from build123d import *

# Parameters (mm, degrees)
SKETCH1_W           = 26.25
SKETCH1_H           = 22
SKETCH1_R           = 3
SKETCH1_R_2         = 13
BOSS_EXTRUDE1_DEPTH = 5
FILLET1_R           = 5
SKETCH2_R           = 1.625
CUT_EXTRUDE1_DEPTH  = 5
CUT_EXTRUDE2_START  = -5
SKETCH3_R           = 1.15
SKETCH3_R_2         = 13
CUT_EXTRUDE2_DEPTH  = 5
SKETCH5_W           = 20
SKETCH5_H           = 3
BOSS_EXTRUDE2_DEPTH = 10
SKETCH6_R           = 1.65
CUT_EXTRUDE4_DEPTH  = 28
CHAMFER1_SIZE       = 10
CHAMFER1_SIZE_2     = 17.320508076
SKETCH9_W           = 20
SKETCH9_H           = 5
CUT_EXTRUDE6_DEPTH  = 5
FILLET3_R           = 5
CUT_EXTRUDE9_START  = -3
CUT_EXTRUDE9_DEPTH  = 3
SKETCH16_W          = 40
SKETCH16_H          = 8
CUT_EXTRUDE11_DEPTH = 10
SKETCH17_W          = 88.86330123
SKETCH17_H          = 4
CUT_EXTRUDE12_DEPTH = 10


# Some blends are built 0.0001 mm under size
with BuildPart() as part:
    # Sketch1 → Boss-Extrude1 (new body)
    # profile 1 of 3: a face of its own
    with BuildSketch(Plane(origin=(0, 0, 0), x_dir=(1, 0, 0), z_dir=(0, 1, 0))):
        with Locations((18.375, 0)):
            Rectangle(SKETCH1_W, SKETCH1_H)
        with Locations(Location((20, 0, 0), (0, 0, 270))):
            Circle(SKETCH1_R, mode=Mode.SUBTRACT)
    # profile 2 of 3: a face of its own
    with BuildSketch(Plane(origin=(0, 0, 0), x_dir=(1, 0, 0), z_dir=(0, 1, 0))):
        with Locations((-18.375, 0)):
            Rectangle(SKETCH1_W, SKETCH1_H)
        with Locations(Location((-20, 0, 0), (0, 0, 270))):
            Circle(SKETCH1_R, mode=Mode.SUBTRACT)
    # profile 3 of 3: a face of its own
    with BuildSketch(Plane(origin=(0, 0, 0), x_dir=(1, 0, 0), z_dir=(0, 1, 0))):
        with BuildLine():
            Line((-5.25, -11), (-31.5, -11))
            Line((-31.5, -11), (-50, -11))
            add(Edge.make_bspline(
                [(-50, -11), (-77.2307176, -35.658609428), (-60, -76)],
                knots=[0, 0, 0, 1, 1, 1], degree=2))
            Line((-60, -76), (-22, -76))
            Line((-22, -76), (-22, -51))
            Line((-22, -51), (22, -51))
            Line((22, -51), (22, -76))
            Line((22, -76), (60, -76))
            add(Edge.make_bspline(
                [(50, -11), (77.2307176, -35.658609428), (60, -76)],
                knots=[0, 0, 0, 1, 1, 1], degree=2))
            Line((50, -11), (31.5, -11))
            Line((31.5, -11), (5.25, -11))
            Line((5.25, -11), (-5.25, -11))
        make_face()
        with Locations(Location((-38, -60, 0), (0, 0, 270))):
            Circle(SKETCH1_R_2, mode=Mode.SUBTRACT)
        with Locations(Location((38, -60, 0), (0, 0, 270))):
            Circle(SKETCH1_R_2, mode=Mode.SUBTRACT)
    extrude(amount=BOSS_EXTRUDE1_DEPTH)

    # Fillet1
    fillet1_edges = [part.edges().sort_by_distance(p)[0] for p in [
        (60, 2.5, 76),
        (-60, 2.5, 76),
    ]]
    fillet(fillet1_edges, radius=FILLET1_R)

    # Sketch2 → Cut-Extrude1 (cut)
    with BuildSketch(Plane(origin=(0, 5, 0), x_dir=(1, 0, 0), z_dir=(0, 1, 0))):
        with Locations(Location((-60, -56, 0), (0, 0, 270))):
            Circle(SKETCH2_R)
        with Locations(Location((60, -56, 0), (0, 0, 270))):
            Circle(SKETCH2_R)
        with Locations(Location((-45, -17, 0), (0, 0, 270))):
            Circle(SKETCH2_R)
        with Locations(Location((-60, -34, 0), (0, 0, 270))):
            Circle(SKETCH2_R)
        with Locations(Location((60, -34, 0), (0, 0, 270))):
            Circle(SKETCH2_R)
        with Locations(Location((45, -17, 0), (0, 0, 270))):
            Circle(SKETCH2_R)
        with Locations(Location((0, -18, 0), (0, 0, 270))):
            Circle(SKETCH2_R)
        with Locations(Location((0, -36, 0), (0, 0, 270))):
            Circle(SKETCH2_R)
    extrude(amount=-CUT_EXTRUDE1_DEPTH, mode=Mode.SUBTRACT)

    # Sketch3 → Cut-Extrude2 (cut)
    with BuildSketch(Plane(origin=(0, 5, 0), x_dir=(1, 0, 0), z_dir=(0, 1, 0)).offset(CUT_EXTRUDE2_START)):
        with Locations(Location((-30, -24, 0), (0, 0, 270))):
            Circle(SKETCH3_R)
        with Locations(Location((-38, -60, 0), (0, 0, 270))):
            Circle(SKETCH3_R_2)
        with Locations(Location((-24.5, -37.5, 0), (0, 0, 270))):
            Circle(SKETCH3_R)
        with Locations(Location((-46, -24, 0), (0, 0, 270))):
            Circle(SKETCH3_R)
        with Locations(Location((-51.5, -37.5, 0), (0, 0, 270))):
            Circle(SKETCH3_R)
        with Locations(Location((24.5, -37.5, 0), (0, 0, 270))):
            Circle(SKETCH3_R)
        with Locations(Location((30, -24, 0), (0, 0, 270))):
            Circle(SKETCH3_R)
        with Locations(Location((46, -24, 0), (0, 0, 270))):
            Circle(SKETCH3_R)
        with Locations(Location((51.5, -37.5, 0), (0, 0, 270))):
            Circle(SKETCH3_R)
    extrude(amount=CUT_EXTRUDE2_DEPTH, mode=Mode.SUBTRACT)

    # Sketch5 → Boss-Extrude2 (add)
    with BuildSketch(Plane(origin=(0, 5, 0), x_dir=(1, 0, 0), z_dir=(0, 1, 0))):
        with Locations((0, -49.5)):
            Rectangle(SKETCH5_W, SKETCH5_H)
    extrude(amount=BOSS_EXTRUDE2_DEPTH)

    # Sketch6 → Cut-Extrude4 (cut)
    with BuildSketch(Plane.XY.offset(76)):
        with Locations((0, 7)):
            Circle(SKETCH6_R)
        with Locations((0, 7.5)):
            Circle(SKETCH6_R)
        with Locations((0, 6.5)):
            Circle(SKETCH6_R)
    extrude(amount=-CUT_EXTRUDE4_DEPTH, mode=Mode.SUBTRACT)

    # Chamfer1
    # the kernel refuses this chamfer: 17.320508076, 10 mm, written as the material it adds along each edge
    with BuildSketch(Plane(origin=(-10, 5, 51), x_dir=(-0.9983227437537926, -0.05789386240267139, 0), z_dir=(0, 0, -1))) as chamfer1_piece_1_section:
        Polygon((CHAMFER1_SIZE * 0.998322743754, CHAMFER1_SIZE * 0.0578938624027), (-CHAMFER1_SIZE_2 * 0.0578938624016, CHAMFER1_SIZE_2 * 0.998322743736), (0, 0), align=None)
    chamfer1_piece_1 = extrude(amount=3, mode=Mode.PRIVATE)
    chamfer1_piece_1 = split(chamfer1_piece_1, bisect_by=Plane(origin=(-13.731694811, 15, 49.5), z_dir=(0, -1, 0)), keep=Keep.TOP, mode=Mode.PRIVATE)
    add(chamfer1_piece_1)
    with BuildSketch(Plane(origin=(10, 5, 48), x_dir=(0.9983227437537926, -0.05789386240267139, 0), z_dir=(0, 0, 1))) as chamfer1_piece_2_section:
        Polygon((CHAMFER1_SIZE * 0.998322743754, CHAMFER1_SIZE * 0.0578938624027), (-CHAMFER1_SIZE_2 * 0.0578938624016, CHAMFER1_SIZE_2 * 0.998322743736), (0, 0), align=None)
    chamfer1_piece_2 = extrude(amount=3, mode=Mode.PRIVATE)
    chamfer1_piece_2 = split(chamfer1_piece_2, bisect_by=Plane(origin=(13.731694811, 15, 49.5), z_dir=(0, -1, 0)), keep=Keep.TOP, mode=Mode.PRIVATE)
    add(chamfer1_piece_2)

    # Sketch9 → Cut-Extrude6 (cut)
    with BuildSketch(Plane(origin=(0, 5, 0), x_dir=(1, 0, 0), z_dir=(0, 1, 0))):
        with Locations((0, -45.5)):
            Rectangle(SKETCH9_W, SKETCH9_H)
    extrude(amount=-CUT_EXTRUDE6_DEPTH, mode=Mode.SUBTRACT)

    # Fillet3
    fillet3_edges = [part.edges().sort_by_distance(p)[0] for p in [
        (-10, 2.5, 43),
        (10, 2.5, 43),
    ]]
    fillet(fillet3_edges, radius=FILLET3_R - 0.0001)  # a hair under: the kernel refuses the full size

    # Sketch8 → Cut-Extrude9 (cut)
    with BuildSketch(Plane(origin=(0, 5, 0), x_dir=(1, 0, 0), z_dir=(0, 1, 0)).offset(CUT_EXTRUDE9_START)):
        with BuildLine():
            Line((-27.5, -27.5), (-48.5, -27.5))
            Line((-48.5, -27.5), (-48.5, -52.335145142))
            ThreePointArc((-48.5, -52.335145142), (-38, -47), (-27.5, -52.335145142))
            Line((-27.5, -52.335145142), (-27.5, -27.5))
        make_face()
        with BuildLine():
            ThreePointArc((27.5, -52.335145142), (38, -47), (48.5, -52.335145142))
            Line((48.5, -52.335145142), (48.5, -27.5))
            Line((48.5, -27.5), (27.5, -27.5))
            Line((27.5, -27.5), (27.5, -52.335145142))
        make_face()
    extrude(amount=CUT_EXTRUDE9_DEPTH, mode=Mode.SUBTRACT)

    # Sketch16 → Cut-Extrude11 (cut)
    with BuildSketch(Plane(origin=(0, 5, 0), x_dir=(1, 0, 0), z_dir=(0, 1, 0))):
        with Locations((0, -26)):
            Rectangle(SKETCH16_W, SKETCH16_H)
    extrude(amount=-CUT_EXTRUDE11_DEPTH, mode=Mode.SUBTRACT)

    # Sketch17 → Cut-Extrude12 (cut)
    with BuildSketch(Plane(origin=(0, 5, 0), x_dir=(1, 0, 0), z_dir=(0, 1, 0))):
        with Locations((-9.103732695, 9)):
            Rectangle(SKETCH17_W, SKETCH17_H)
    extrude(amount=-CUT_EXTRUDE12_DEPTH, mode=Mode.SUBTRACT)


solid = part.part
Design review of the part built by this model. Coordinates are the model's own, in mm. A direction names the side the tool comes from. Round coordinates to 2 decimals unless told otherwise and drop trailing zeros. Order: outer loops, then holes, each group sorted by start corner. A loop starts at its lowest first (then second) coordinate and runs counter-clockwise, first axis right, second up.
1) Consider section A-A (z = 0). State the section outline as (x, y) points, plus the area to 4 significant figures.
The answers:
outline: (-31.5, 0) - (-23, 0) - (-23, 5) - (-31.5, 5) - close; (-17, 0) - (-5.25, 0) - (-5.25, 5) - (-17, 5) - close; (5.25, 0) - (17, 0) - (17, 5) - (5.25, 5) - close; (23, 0) - (31.5, 0) - (31.5, 5) - (23, 5) - close
area: 202.5 mm2
2) Consider section D-D (z = 56). Count the separate pieces of the cut face and the enclosed holes in it, plus the area to 3 significant figures.
The answers:
separate pieces: 6
enclosed holes: 0
area: 160 mm2
3) Machinability: for faces 5 (the flat face through (22, 2, 63)), 6 (the flat face through (-5.25, 2, 2)), 7 (the flat face through (0, 10, 48)), which of the approach directions +Z, -Z, +X, -X, +Y, -Y give a long, thin tool a straight path to every point of the face, cutting with its end or side? Answer none if there is none.
The answers:
face 5: +Z, +Y, -Y
face 6: -Z, +Y, -Y
face 7: +Y
4) Consider section B-B (x = -34.5). State the section outline as (y, z) points, plus the area to 3 significant figures.
The answers:
outline: (0, 11) - (5, 11) - (5, 27.5) - (2, 27.5) - (2, 47.48) - (0, 47.48) - close; (0, 72.52) - (5, 72.52) - (5, 76) - (0, 76) - close
area: 140 mm2
5) Consider section C-C (y = 11.5). State the section outline as (x, z) points, plus the area to 3 significant figures.
The answers:
outline: (-16.25, 48) - (16.25, 48) - (16.25, 51) - (-16.25, 51) - close
area: 97.5 mm2
6) Clearance check with flat-ended pins moving along their axes: pin 1 Ø1.5 at (y, z) = (2, 5) entering from +X; pin 2 Ø1.5 at (y, z) = (2, 25) entering from -X; pin 3 Ø5 at (x, z) = (31, 56) entering from -Y; pin 4 Ø12 at (x, z) = (-32, 32) entering from +Y. State where each tip first meets the part, or that it passes through.
The answers:
pin 1: stops at x = 31.5
pin 2: stops at x = -61.62
pin 3: passes through
pin 4: stops at y = 5
7) For L1, parallel to X at y = 2.85, z = 0; L2, parallel to X at y = 1.55, z = 17 (3 decimals); L3, parallel to Z at x = -38, y = 2.1, list the stretches that pass through material, from the lowest coordinate up.
The answers:
L1: x = -31.5 to -23, -17 to -5.25, 5.25 to 17, 23 to 31.5
L2: x = -55.776 to -46.625, -43.375 to -1.281, 1.281 to 43.375, 46.625 to 55.776
L3: z = 11 to 27.5, 73 to 76
8) Draft analysis for pull direction X (two halves, no side actions). For faces 1 (the flat face through (-19, 3, -7)), 2 (the flat face through (31.5, 2, 2)), 3 (the flat face through (-17.154, 9.93, 49.521)), 4 (the cylindrical face through (-0.04, 4.85, 49.52)), state which applies: released by +X, released by -X, zero draft, split by the parting line, or undercut.
The answers:
face 1: zero draft
face 2: released by +X
face 3: released by -X
face 4: undercut
